Here's how the part is built. I have some questions about the finished solid (model axes, mm). Face numbers are marked on the shaded views. Coordinates: 2 decimals unless noted, no trailing zeros. Write each loop counter-clockwise with the first axis right and the second up, starting at its lowest first coordinate (ties: lowest second). Pieces come first, ordered by that corner, then holes.
from build123d import *

# Parameters (mm, degrees)
SKETCH1_W           = 400
SKETCH1_H           = 250
BOSS_EXTRUDE1_DEPTH = 20
SKETCH2_W           = 40
SKETCH2_H           = 40
SKETCH2_R           = 10
BOSS_EXTRUDE2_DEPTH = 30


with BuildPart() as part:
    # Sketch1 → Boss-Extrude1 (new body)
    with BuildSketch(Plane(origin=(0, 0, 0), x_dir=(1, 0, 0), z_dir=(0, 1, 0))):
        Rectangle(SKETCH1_W, SKETCH1_H)
    extrude(amount=BOSS_EXTRUDE1_DEPTH)

    # Sketch2 → Boss-Extrude2 (add)
    with BuildSketch(Plane.XY.offset(125)):
        with Locations((-180, 40)):
            Rectangle(SKETCH2_W, SKETCH2_H)
        with Locations((-180, 40)):
            Circle(SKETCH2_R, mode=Mode.SUBTRACT)
        with Locations((180, 40)):
            Rectangle(SKETCH2_W, SKETCH2_H)
        with Locations((180, 40)):
            Circle(SKETCH2_R, mode=Mode.SUBTRACT)
    boss_extrude2 = extrude(amount=-BOSS_EXTRUDE2_DEPTH)

    # Mirror1: Boss-Extrude2 across plane
    add(boss_extrude2.mirror(Plane.XY))


solid = part.part
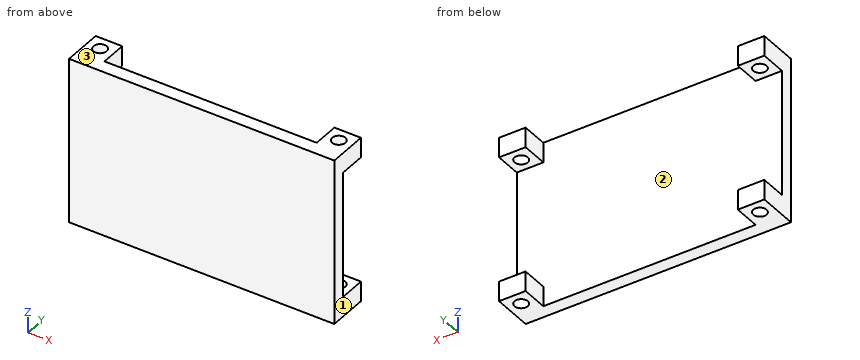
1. If I drill on line 1 (Y direction, x = 180, z = 105.5); line 2 (Z direction, x = -168, y = 41); line 3 (X direction, y = 25.5, z = -109.5), over which ranges is the centre line in solid material (lowest first)?
2. For pin 1 Ø18 at (x, y) = (180, 40) entering from -Z, with a flat end and sliding along its axis, tell me the tip position at first contact or that it passes through.
3. I want a section at C-C (x = -180). List the corners of the cut face in (y, z) for me, then the cut area to 3 significant figures.
4. Thinking about a two-plate mould opening in X: for the marked faces 1, 2 and 3, which applies, pulls with the +X half, pulls with the -X half, needs draft (parallel to the pull), parting line crosses it, or undercut?
5. I want a section at B-B (z = 102). List the corners of the cut face in (x, y) for me.
6. I want a section at A-A (y = 26). List the corners of the cut face in (x, z) for me.
7. I want a section at D-D (z = -36). List the corners of the cut face in (x, y) for me, then the cut area to 3 significant figures.
Response values:
1. line 1: y = 0 to 30, 50 to 60
1. line 2: z = -125 to -95, 95 to 125
1. line 3: x = -200 to -160, 160 to 200
2. pin 1: passes through
3. outline: (0, -125) - (30, -125) - (30, -95) - (20, -95) - (20, 95) - (30, 95) - (30, 125) - (0, 125) - close; (50, -125) - (60, -125) - (60, -95) - (50, -95) - close; (50, 95) - (60, 95) - (60, 125) - (50, 125) - close
3. area: 6,200 mm2
4. face 1: pulls with the +X half
4. face 2: undercut
4. face 3: needs draft
5. outline: (-200, 0) - (200, 0) - (200, 60) - (160, 60) - (160, 20) - (-160, 20) - (-160, 60) - (-200, 60) - close; hole circle Ø20 at (-180, 40); hole circle Ø20 at (180, 40)
6. outline: (-200, -125) - (-160, -125) - (-160, -95) - (-200, -95) - close; (-200, 95) - (-160, 95) - (-160, 125) - (-200, 125) - close; (160, -125) - (200, -125) - (200, -95) - (160, -95) - close; (160, 95) - (200, 95) - (200, 125) - (160, 125) - close
7. outline: (-200, 0) - (200, 0) - (200, 20) - (-200, 20) - close
7. area: 8,000 mm2
